Job drawing, mm, ordinate dimensions from the low corner. One solid piece. Give positions to 0.01 mm unless a question says otherwise; leave off trailing zeros. Order: outer loops, then holes, each group sorted by start corner. A loop starts at its lowest first (then second) coordinate and runs counter-clockwise, first axis right, second up.
1. Slice it at C-C on x = 26. List the corners of the cut face in (y, z), and give its area (3 significant figures).
2. Slice it at B-B on z = 61.5. List the corners of the cut face in (x, y).
3. Slice it at D-D on z = 12. List the corners of the cut face in (x, y), and give its area (3 significant figures).
4. Drop flat-ended pins along their axis: pin 1 Ø8 at (x, z) = (19, 61.5) entering from +Y; pin 2 Ø10 at (x, z) = (26.5, 66) entering from -Y; pin 3 Ø10 at (y, z) = (10.5, 49.5) entering from +X. Give the stop position or say it passes through.
5. Mould opens along X. For the marked faces 1, 2, 3 and 4 say: +X half, -X half, draft (parallel to the pull), parting line (faces both ways), or undercut.
6. Slice it at A-A on y = 2. List the corners of the cut face in (x, z).
7. Probe line 1 (X direction, y = 2.5, z = 38.5); line 2 (Y direction, x = 4.5, z = 63.5); line 3 (Y direction, x = 28, z = 59.5). List the from-to ranges inside material, lowest first.
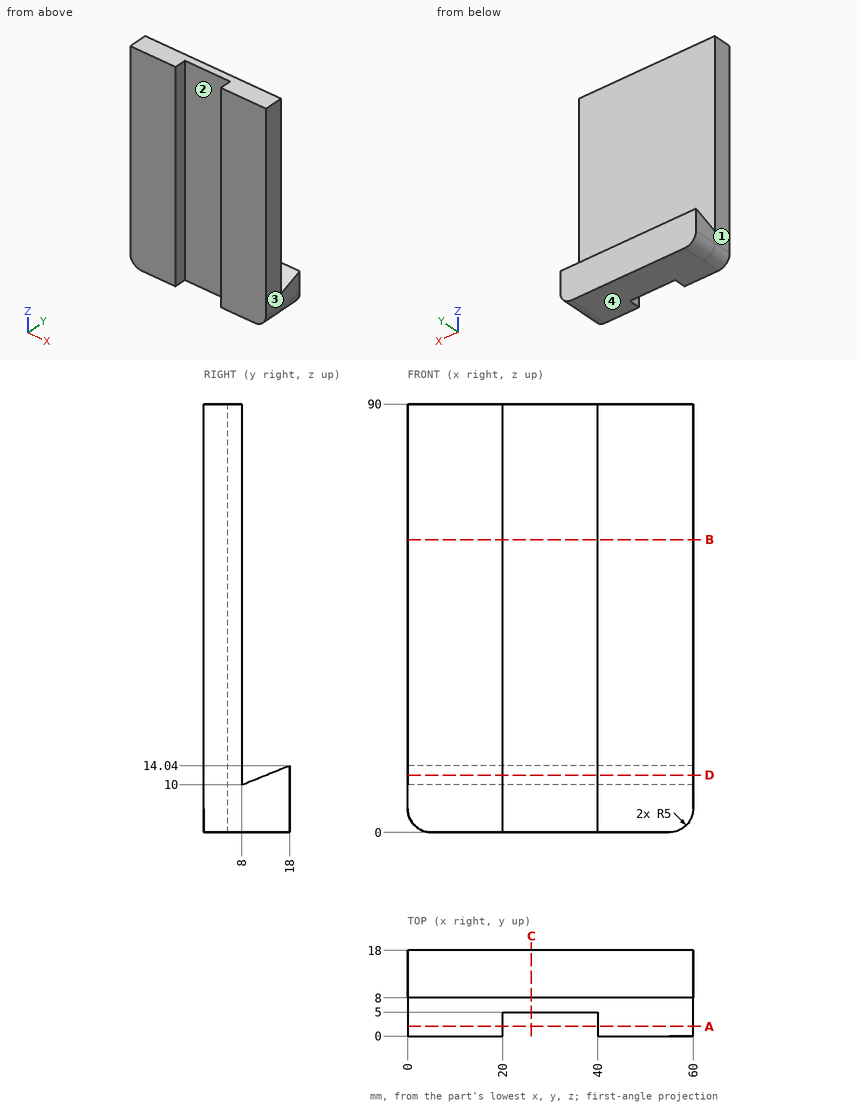
Data:
1. outline: (5, 0) - (18, 0) - (18, 14.04) - (8, 10) - (8, 90) - (5, 90) - close
1. area: 390 mm2
2. outline: (0, 0) - (20, 0) - (20, 5) - (40, 5) - (40, 0) - (60, 0) - (60, 8) - (0, 8) - close
3. outline: (0, 0) - (20, 0) - (20, 5) - (40, 5) - (40, 0) - (60, 0) - (60, 8) - (0, 8) - close; (0, 12.95) - (60, 12.95) - (60, 18) - (0, 18) - close
3. area: 683 mm2
4. pin 1: stops at y = 8
4. pin 2: stops at y = 5
4. pin 3: stops at x = 60
5. face 1: -X half
5. face 2: undercut
5. face 3: +X half
5. face 4: draft
6. outline: (0, 5) arc R5 ccw to (5, 0) - (20, 0) - (20, 90) - (0, 90) - close; (40, 0) - (55, 0) arc R5 ccw to (60, 5) - (60, 90) - (40, 90) - close
7. line 1: x = 0 to 20, 40 to 60
7. line 2: y = 0 to 8
7. line 3: y = 5 to 8
